Geometry check sheet. Reference: the model listing, model coordinates, mm. Face numbers are marked on the shaded views. A direction names the side the tool comes from. Round coordinates to 2 decimals unless told otherwise and drop trailing zeros. Order: outer loops, then holes, each group sorted by start corner. A loop starts at its lowest first (then second) coordinate and runs counter-clockwise, first axis right, second up. Notation, with made-up numbers: (12, 36.5) - (38, 36.5) arc R35 ccw to (38, 71.5) - close; hole circle Ø2 at (49.5, 37.5). An arc over 180 degrees is marked (long way). Answer as CSV lines item,"result". Start each with the question number.
```python
from build123d import *

# Parameters (mm, degrees)
F1_DEPTH  = 20
F3_DEPTH  = 4
F5_DEPTH  = 1
F7_DEPTH  = 20.001
F10_W     = 15
F10_H     = 9.1
F11_DEPTH = 1
F12_D     = 5.55752


# Not quite as in the source:
# - a pattern or mirror of a feature is missing from the dataset's text; its kind, count and spacing are read off the source's solid


with BuildPart() as f1:
    # F0 (on Front) → F1 (new body)
    with BuildSketch(Plane.XZ):
        Polygon((-16.45, 3), (-19.25, -1.7), (-18.09, -1.7), (-17.0772340426, 0), (0, 0), (0, 3), align=None)
    extrude(amount=F1_DEPTH)

    # F2 (on face) → F3 (cut)
    with BuildSketch(Plane.XZ.offset(20)):
        Polygon((-16.2, 2), (-0.5, 2), (0, 1.8180148829), (0, 3), (-16, 3), (-16.5, 2.1091910703), align=None)
    f3 = extrude(amount=-F3_DEPTH, mode=Mode.SUBTRACT)

    # F3_copies: F3 across plane
    add(f3.mirror(Plane.ZX.offset(-10)), mode=Mode.SUBTRACT)

    # F4 (on face) → F5 (cut)
    with BuildSketch(Plane.XZ.offset(20)):
        Polygon((0, 0), (0, 1.8180148829), (-0.5, 2), (-16.2, 2), (-16.5, 2.1091910703), (-17.683862779, 0), align=None)
    f5 = extrude(amount=-F5_DEPTH, mode=Mode.SUBTRACT)

    # F5_copies: F5 across plane
    add(f5.mirror(Plane.ZX.offset(-10)), mode=Mode.SUBTRACT)

    # F6 (on face) → F7 (cut, through all)
    with BuildSketch(Plane.XZ.offset(20)):
        Polygon((-18.67, -1.7), (-18.09, -1.7), (-17.0772340426, 0), (-17.683862779, 0), align=None)
    extrude(amount=-F7_DEPTH, mode=Mode.SUBTRACT)

    # F10 (on face) → F11 (cut)
    with BuildSketch(Plane(origin=(0, 0, 0), x_dir=(1, 0, 0), z_dir=(0, 0, -1))):
        with Locations((-9, 10)):
            Rectangle(F10_W, F10_H)
    extrude(amount=-F11_DEPTH, mode=Mode.SUBTRACT)

    # F12 (through all)
    with Locations(Plane.XY.offset(3)):
        with Locations((-8.225, -10)):
            Hole(F12_D / 2)


solid = f1.part
```
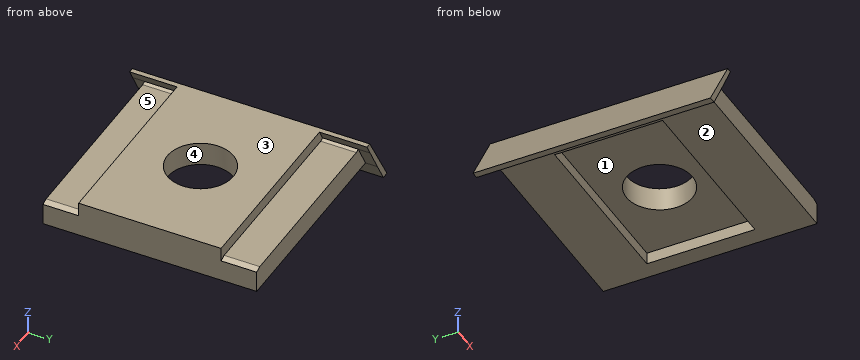
1. Section check B-B on x = -2.75. Record the boundary of the cut face in (y, z), plus the area to 3 significant figures.
2. Go/stop test with flat-tipped pins: pin 1 Ø10 at (x, y) = (-8, -9) entering from -Z; pin 2 Ø1 at (y, z) = (-3, -0.5) entering from -X; pin 3 Ø0.6 at (x, z) = (-8.5, 1) entering from -Y. Record where each tip stops, or that it passes through.
3. Section check C-C on x = -6.25. Record the boundary of the cut face in (y, z), plus the area to 3 significant figures.
4. Access from +Z, -Z, +X, -X, +Y, -Y to the whole of each face (thin tool, end or side, straight path). Record for the marked faces 1, 2 and 3.
5. Section check A-A on y = -10. Record the boundary of the cut face in (x, z), plus the area to 3 significant figures.
6. Section check D-D on y = -6.25. Record the boundary of the cut face in (x, z), plus the area to 3 significant figures.
7. Thickness scan on probe 1 along Y at (x, z) = (-7.75, 0.5); probe 2 along Z at (x, y) = (-3.5, -3.25); probe 3 along Z at (x, y) = (-8.5, -13.5). Record the ranges inside material, lowest first.
8. Draft check along Y on the marked faces 4 and 5. Enter one of: released by +Y, released by -Y, zero draft, split by the parting line, or undercut.
Numbers:
1,outline,"(-19, 0) - (-14.55, 0) - (-14.55, 1) - (-5.45, 1) - (-5.45, 0) - (-1, 0) - (-1, 2) - (-4, 2) - (-4, 3) - (-16, 3) - (-16, 2) - (-19, 2) - close"
1,area,"38.9 mm2"
2,pin 1,"stops at z = 0"
2,pin 2,"stops at x = -18.83"
2,pin 3,"stops at y = -19"
3,outline,"(-19, 0) - (-14.55, 0) - (-14.55, 1) - (-11.95, 1) - (-11.95, 3) - (-16, 3) - (-16, 2) - (-19, 2) - close; (-8.05, 1) - (-5.45, 1) - (-5.45, 0) - (-1, 0) - (-1, 2) - (-4, 2) - (-4, 3) - (-8.05, 3) - close"
3,area,"31.1 mm2"
4,face 1,"-Z"
4,face 2,"-Z, +X, +Y, -Y"
4,face 3,"+Z, +X, -X, +Y, -Y"
5,outline,"(-19.25, -1.7) - (-18.67, -1.7) - (-17.68, 0) - (-16.5, 0) - (-16.5, 1) - (-11, 1) - (-11, 3) - (-16.45, 3) - close; (-5.45, 1) - (-1.5, 1) - (-1.5, 0) - (0, 0) - (0, 3) - (-5.45, 3) - close"
5,area,"26.9 mm2"
6,outline,"(-19.25, -1.7) - (-18.67, -1.7) - (-17.68, 0) - (-16.5, 0) - (-16.5, 1) - (-1.5, 1) - (-1.5, 0) - (0, 0) - (0, 3) - (-16.45, 3) - close"
6,area,"38.0 mm2"
7,probe 1,"y = -19 to -14.55, -5.45 to -1"
7,probe 2,"z = 0 to 2"
7,probe 3,"z = 1 to 3"
8,face 4,"undercut"
8,face 5,"zero draft"
